```python
from build123d import *

# Parameters (mm, degrees)
SKETCH1_R           = 19.05
SKETCH1_R_2         = 6.35
BOSS_EXTRUDE1_DEPTH = 31.75
SKETCH2_R           = 4.25
CUT_EXTRUDE1_DEPTH  = 20.05
SKETCH2_6_R         = 2.5
CUT_EXTRUDE3_DEPTH  = 20.0500001
CHAMFER1_SIZE       = 0.508


with BuildPart() as part:
    # Sketch1 → Boss-Extrude1 (new body)
    with BuildSketch(Plane(origin=(0, 0, 0), x_dir=(0, 0, -1), z_dir=(1, 0, 0))):
        Circle(SKETCH1_R)
        Circle(SKETCH1_R_2, mode=Mode.SUBTRACT)
    extrude(amount=BOSS_EXTRUDE1_DEPTH)

    # Sketch2 → Cut-Extrude1 (cut, through all)
    with BuildSketch(Plane.XY):
        with Locations((15.875, 0)):
            Circle(SKETCH2_R)
    extrude(amount=CUT_EXTRUDE1_DEPTH, mode=Mode.SUBTRACT)

    # Sketch2<6> → Cut-Extrude3 (cut, through all)
    with BuildSketch(Plane.XY):
        with Locations((15.875, 0)):
            Circle(SKETCH2_6_R)
    extrude(amount=-CUT_EXTRUDE3_DEPTH, mode=Mode.SUBTRACT)

    # Chamfer1
    chamfer1_edges = [part.edges().sort_by_distance(p)[0] for p in [
        (0, 0, 19.05),
        (31.75, 0, 19.05),
    ]]
    chamfer(chamfer1_edges, length=CHAMFER1_SIZE)


solid = part.part
```
Input: part model. Units: mm. Frame: model coordinates. A direction names the side the tool comes from. Round coordinates to 2 decimals unless told otherwise and drop trailing zeros. Loops run counter-clockwise (first coordinate to the right, second up) from the corner with the lowest first, then second, coordinate; pieces in that order, holes last. Notation, with made-up numbers: M 82.5,7.5 L 126.5,7.5 A20 cw 126.5,41.5 Z; hole C 55.25,9.25 d9. An arc over 180 degrees is marked long. Answer in a Markdown table with one row per item. Add a question column.
1. Mould query, pull axis Y, two halves, no side actions, for faces 3 (the face through (15.66, 5.72, -18.17)), 4 (the face through (15.653, 5.354, -3.414)), 5 (the face through (0, -8, 0)). Classes: released by +Y, released by -Y, zero draft, split by the parting line, or undercut.
2. Set-up query: faces 1 (the face through (19.8, -1.63, 11.78)), 2 (the face through (13.377, 0.11, -12.351)). Return all of +Z, -Z, +X, -X, +Y, -Y with unobstructed straight access to the full face (end or side cutting, diameter ignored); none if empty.
3. Contact query for flat-ended pins moving along their axis: pin 1 (2 mm diameter, centred on x = 17, z = -12.5, fed in from +Y); pin 2 (4 mm diameter, centred on x = 17.5, y = -11.5, fed in from -Z); pin 3 (5 mm diameter, centred on x = 27.5, y = 14.5, fed in from -Z). Output: stop coordinate, or through.
4. Section C-C (x = 6). Output: boundary loops of the cut face in (y, z), and give its area (3 significant figures).
5. Section D-D (x = 19). Output: boundary loops of the cut face in (y, z).
6. Section A-A (y = 0). Output: boundary loops of the cut face in (x, z) (3 decimals).
7. Section B-B (z = 0). Output: boundary loops of the cut face in (x, y), and give its area (3 significant figures).
8. Ray query, probe 1 along X at (y, z) = (0, -15.5) (3 decimals); probe 2 along Y at (x, z) = (21.5, 0); probe 3 along Z at (x, y) = (28, 4.5). Return the intervals inside material, ascending.
Values follow:
| question | item | result |
|---|---|---|
| 1 | face 3 | split by the parting line |
| 1 | face 4 | undercut |
| 1 | face 5 | zero draft |
| 2 | face 1 | +Z |
| 2 | face 2 | +Z, -Z |
| 3 | pin 1 | y = 15.19 |
| 3 | pin 2 | z = -16.51 |
| 3 | pin 3 | z = -14.8 |
| 4 | outline | C 0,0 d38.1; hole C 0,0 d12.7 |
| 4 | area | 1,010 mm^2 |
| 5 | outline | M -2.88,5.66 L -2.88,18.83 A19.05 ccw long 2.88,18.83 L 2.88,5.66 A6.35 cw long Z |
| 6 | outline | M 0,-18.542 L 0.508,-19.05 L 13.375,-19.05 L 13.375,-6.35 L 0,-6.35 Z; M 0,6.35 L 11.625,6.35 L 11.625,19.05 L 0.508,19.05 L 0,18.542 Z; M 18.375,-19.05 L 31.242,-19.05 L 31.75,-18.542 L 31.75,-6.35 L 18.375,-6.35 Z; M 20.125,6.35 L 31.75,6.35 L 31.75,18.542 L 31.242,19.05 L 20.125,19.05 Z |
| 7 | outline | M 0,-18.54 L 0.51,-19.05 L 31.24,-19.05 L 31.75,-18.54 L 31.75,-6.35 L 0,-6.35 Z; M 0,6.35 L 31.75,6.35 L 31.75,18.54 L 31.24,19.05 L 0.51,19.05 L 0,18.54 Z |
| 7 | area | 806 mm^2 |
| 8 | probe 1 | 0 to 13.375, 18.375 to 31.75 |
| 8 | probe 2 | -19.05 to -6.35, 6.35 to 19.05 |
| 8 | probe 3 | -18.51 to -4.48, 4.48 to 18.51 |
